Here's how the part is built. I have some questions about the finished solid (model axes, mm). Give positions to 0.01 mm unless a question says otherwise; leave off trailing zeros. Loops run counter-clockwise (first coordinate to the right, second up) from the corner with the lowest first, then second, coordinate; pieces in that order, holes last. Notation, with made-up numbers: (26.5, 64.25) - (77.5, 64.25) arc R25 cw to (77.5, 88.25) - close; hole circle Ø1 at (-13, 26). An arc over 180 degrees is marked (long way). Use a Markdown table: item, result.
from build123d import *

# Parameters (mm, degrees)
BOSS_EXTRUDE1_DEPTH = 500


with BuildPart() as part:
    # Sketch1 → Boss-Extrude1 (new body)
    with BuildSketch(Plane(origin=(0, 0, 0), x_dir=(0, 0, -1), z_dir=(1, 0, 0))):
        with BuildLine():
            Line((38.1, 1000), (101.4671252, 275.710444691))
            ThreePointArc((101.4671252, 275.710444691), (172.142788026, 115.087782586), (325.99444252, 30.681874577))
            Line((325.99444252, 30.681874577), (500, 0))
            Line((500, 0), (0, 0))
            Line((0, 0), (0, 1000))
            Line((0, 1000), (38.1, 1000))
        make_face()
    extrude(amount=-BOSS_EXTRUDE1_DEPTH)


solid = part.part
(1) Will these pins go through, and if not, where does the flat tip stop? pin 1 (2 mm diameter, centred on x = -393.5, y = 583, fed in from -Z); pin 2 (10 mm diameter, centred on x = -329.5, y = 247.5, fed in from -Z); pin 3 (6 mm diameter, centred on x = -121, y = 489, fed in from -Z).
A:
| item | result |
|---|---|
| pin 1 | z = -74.67 |
| pin 2 | z = -106.45 |
| pin 3 | z = -83.07 |
(2) Suppose I cut it at C-C on z = -147. Write out the boundary of the cut face in (x, y), plus the area to 3 significant figures.
A:
| item | result |
|---|---|
| outline | (-500, 0) - (0, 0) - (0, 147) - (-500, 147) - close |
| area | 73,500 mm2 |
(3) Suppose I cut it at A-A on x = -317. Write out the boundary of the cut face in (y, z), plus the area to 3 significant figures.
A:
| item | result |
|---|---|
| outline | (0, -500) - (30.68, -325.99) arc R272.97 cw to (275.71, -101.47) - (1000, -38.1) - (1000, 0) - (0, 0) - close |
| area | 103,000 mm2 |
(4) If I drill on line 1 (Z direction, x = -35.5, y = 729); line 2 (Y direction, x = -100, z = -299.5); line 3 (Z direction, x = -274.5, y = 380), over which ranges is the centre line in solid material (lowest first)?
A:
| item | result |
|---|---|
| line 1 | -61.81 to 0 |
| line 2 | 0 to 36.73 |
| line 3 | -92.34 to 0 |
(5) Suppose I cut it at B-B on y = 121. Write out the boundary of the cut face in (x, z).
A:
| item | result |
|---|---|
| outline | (-500, -166.88) - (0, -166.88) - (0, 0) - (-500, 0) - close |
